Here's how the part is built. I have some questions about the finished solid (model axes, mm). Round coordinates to 2 decimals unless told otherwise and drop trailing zeros. Write each loop counter-clockwise with the first axis right and the second up, starting at its lowest first coordinate (ties: lowest second). Pieces come first, ordered by that corner, then holes. Notation, with made-up numbers: M -29.75,-11.5 L -6.75,-11.5 A37 cw -6.75,25.5 Z; hole C 76.5,-24 d7. An arc over 180 degrees is marked long. Use one line per item in the form item = value. Start each with the question number.
Q1. I need wall thicknesses on line 1 along X through (y, z) = (-3.25, 0); line 2 along Z through (x, y) = (3, -11.75); line 3 along Z through (x, y) = (-4.5, -14.75). Which ranges of each line are inside material? Lowest first, please. Write a range as from..to.
Q2. I want a section at A-A on y = -6. List the corners of the cut face in (x, z) for me.
Q3. I want a section at B-B on z = 0. List the corners of the cut face in (x, y) for me.
Q4. I'm going to push flat-ended pins straight in: pin 1 Ø1.5 at (x, y) = (9.5, -13) entering from +Z; pin 2 Ø4 at (y, z) = (-6.5, 11) entering from +X; pin 3 Ø5 at (x, y) = (-1, -11) entering from -Z; pin 4 Ø5 at (x, z) = (-3, 1.5) entering from +Y. Where does each tip first touch, or does it pass through?
Q5. We'd pull the mould along Z, two halves only. Please class faces 1 (the face through (-7.81, -8.11, 1.73)), 2 (the face through (-12.304, -15.904, 7.14)), 3 (the face through (12.304, -0.096, -7.14)), 4 (the face through (-13.856, -8, 0)): +Z half, -Z half, draft (parallel to the pull), parting line (faces both ways), or undercut.
```python
from build123d import *

# Parameters (mm, degrees)
BOSS_EXTRUDE2_DEPTH = 16
SKETCH9_R           = 8
CUT_EXTRUDE3_DEPTH  = 64


with BuildPart() as part:
    # Sketch4 → Boss-Extrude2 (new body)
    with BuildSketch(Plane(origin=(0, 0, 0), x_dir=(1, 0, 0), z_dir=(0, 1, 0))):
        Polygon((0, -16), (13.856406461, -8), (13.856406461, 8), (0, 16), (-13.856406461, 8), (-13.856406461, -8), align=None)
    extrude(amount=-BOSS_EXTRUDE2_DEPTH)

    # Sketch5 → Cut-Revolve2 (revolve, cut)
    with BuildSketch(Plane.XY):
        Polygon((-13.875900938, 0), (-18.013042907, 0), (-18.013042907, -1.135273282), align=None)
    cut_revolve2 = revolve(axis=Axis((0, 7.032369226, 0), (0, -1, 0)), mode=Mode.SUBTRACT)

    # Sketch9 → Cut-Extrude3 (cut)
    with BuildSketch(Plane.XZ.offset(16)):
        with Locations(Location((0, 0, 0), (0, 0, 270))):
            Circle(SKETCH9_R)
    extrude(amount=-CUT_EXTRUDE3_DEPTH, mode=Mode.SUBTRACT)

    # Mirror1: Cut-Revolve2 across plane
    add(cut_revolve2.mirror(Plane.ZX.offset(-8)), mode=Mode.SUBTRACT)


solid = part.part
```
Reported:
q1.line_1 = -13.86..-8, 8..13.86
q1.line_2 = -14.27..-7.42, 7.42..14.27
q1.line_3 = -13.4..-6.61, 6.61..13.4
q2.outline = M -13.86,-8 L 0,-16 L 13.86,-8 L 13.86,8 L 0,16 L -13.86,8 Z; hole C 0,0 d16
q3.outline = M -13.86,-16 L -8,-16 L -8,0 L -13.86,0 Z; M 8,-16 L 13.86,-16 L 13.86,0 L 8,0 Z
q4.pin_1 = 10.95
q4.pin_2 = 12.12
q4.pin_3 = -16
q4.pin_4 = through
q5.face_1 = undercut
q5.face_2 = +Z half
q5.face_3 = -Z half
q5.face_4 = draft
